For this review, take the finished solid that the model builds, in its own axes (mm). A direction names the side the tool comes from. Coordinates: 2 decimals unless noted, no trailing zeros. Write each loop counter-clockwise with the first axis right and the second up, starting at its lowest first coordinate (ties: lowest second). Pieces come first, ordered by that corner, then holes.
```python
from build123d import *

# Parameters (mm, degrees)
SKETCH_W             = 162
SKETCH_H             = 37
PAD_DEPTH            = 16
POCKET_DEPTH         = 18.501
POCKET_DEPTH_BACK    = -18.501
POCKET001_DEPTH      = 18.501
POCKET001_DEPTH_BACK = -18.501
POCKET002_DEPTH      = 18.501
POCKET002_DEPTH_BACK = -18.501
POCKET003_DEPTH      = 18.501
POCKET003_DEPTH_BACK = -18.501
POCKET004_DEPTH      = 18.501
POCKET004_DEPTH_BACK = -18.501
SKETCH004_W          = 31.24
SKETCH004_H          = 3.92
POCKET005_DEPTH      = 81.001
POCKET005_DEPTH_BACK = -81.001
SKETCH005_W          = 33.24
SKETCH005_H          = 1
POCKET006_DEPTH      = 81.001
POCKET006_DEPTH_BACK = -81.001


with BuildPart() as part:
    # Sketch → Pad (new body)
    with BuildSketch(Plane.XY):
        Rectangle(SKETCH_W, SKETCH_H)
    extrude(amount=PAD_DEPTH)

    # Sketch001 → Pocket (cut, two sides)
    with BuildSketch(Plane.XZ) as pocket_sk:
        Polygon((81, 16), (81, 9.14), (65, 9.14), (65, -1.45), (83.75, -1.45), (83.75, 16), align=None)
    extrude(amount=-POCKET_DEPTH, mode=Mode.SUBTRACT)
    extrude(pocket_sk.sketch, amount=-POCKET_DEPTH_BACK, mode=Mode.SUBTRACT)

    # MirroredSketch → Pocket001 (cut, two sides)
    with BuildSketch(Plane.XZ) as pocket001_sk:
        Polygon((-81, 16), (-81, 9.14), (-65, 9.14), (-65, -1.45), (-83.75, -1.45), (-83.75, 16), align=None)
    extrude(amount=-POCKET001_DEPTH, mode=Mode.SUBTRACT)
    extrude(pocket001_sk.sketch, amount=-POCKET001_DEPTH_BACK, mode=Mode.SUBTRACT)

    # Sketch002 → Pocket002 (cut, two sides)
    with BuildSketch(Plane.XZ) as pocket002_sk:
        with BuildLine():
            Line((57.5, 3.58), (57.5, -2.6))
            Line((57.5, -2.6), (46.5, -2.6))
            Line((46.5, -2.6), (46.5, 3.58))
            ThreePointArc((57.5, 3.58), (52, 9.08), (46.5, 3.58))
        make_face()
    extrude(amount=-POCKET002_DEPTH, mode=Mode.SUBTRACT)
    extrude(pocket002_sk.sketch, amount=-POCKET002_DEPTH_BACK, mode=Mode.SUBTRACT)

    # MirroredSketch001 → Pocket003 (cut, two sides)
    with BuildSketch(Plane.XZ) as pocket003_sk:
        with BuildLine():
            Line((-57.5, 3.58), (-57.5, -2.6))
            Line((-57.5, -2.6), (-46.5, -2.6))
            Line((-46.5, -2.6), (-46.5, 3.58))
            ThreePointArc((-46.5, 3.58), (-52, 9.08), (-57.5, 3.58))
        make_face()
    extrude(amount=-POCKET003_DEPTH, mode=Mode.SUBTRACT)
    extrude(pocket003_sk.sketch, amount=-POCKET003_DEPTH_BACK, mode=Mode.SUBTRACT)

    # Sketch003 → Pocket004 (cut, two sides)
    with BuildSketch(Plane.XZ) as pocket004_sk:
        with BuildLine():
            Line((-40.2, 4.78), (-40.2, -1.94))
            Line((-40.2, -1.94), (40.2, -1.94))
            Line((40.2, -1.94), (40.2, 4.78))
            ThreePointArc((40.2, 4.78), (39.707939, 5.967939), (38.52, 6.46))
            Line((38.52, 6.46), (-38.52, 6.46))
            ThreePointArc((-38.52, 6.46), (-39.707939, 5.967939), (-40.2, 4.78))
        make_face()
    extrude(amount=-POCKET004_DEPTH, mode=Mode.SUBTRACT)
    extrude(pocket004_sk.sketch, amount=-POCKET004_DEPTH_BACK, mode=Mode.SUBTRACT)

    # Sketch004 → Pocket005 (cut, two sides)
    with BuildSketch(Plane.YZ) as pocket005_sk:
        with Locations((0, 15.32)):
            Rectangle(SKETCH004_W, SKETCH004_H)
    extrude(amount=-POCKET005_DEPTH, mode=Mode.SUBTRACT)
    extrude(pocket005_sk.sketch, amount=-POCKET005_DEPTH_BACK, mode=Mode.SUBTRACT)

    # Sketch005 → Pocket006 (cut, two sides)
    with BuildSketch(Plane.YZ) as pocket006_sk:
        with Locations((0, 13.86)):
            Rectangle(SKETCH005_W, SKETCH005_H)
    extrude(amount=-POCKET006_DEPTH, mode=Mode.SUBTRACT)
    extrude(pocket006_sk.sketch, amount=-POCKET006_DEPTH_BACK, mode=Mode.SUBTRACT)


solid = part.part
```
Q1. Tool access review of faces 1 (the flat face through (-73, 0, 9.14)), 2 (the flat face through (65, 0, 5)), 3 (the flat face through (-1, -17, 16)), 4 (the flat face through (43, 0, 0)), 5 (the flat face through (-57.5, 0, 2)): name each direction out of +Z, -Z, +X, -X, +Y, -Y from which nothing blocks a thin tool from reaching the whole face with its end or side.
Ans:
face 1: -Z, -X, +Y, -Y
face 2: -Z, +X, +Y, -Y
face 3: +Z, +X, -X, +Y, -Y
face 4: -Z, +X, -X, +Y, -Y
face 5: -Z, +Y, -Y
Q2. Add section B-B (y = -7.5). State the section outline as (x, z) points, then the cut area to 3 significant figures.
Ans:
outline: (-81, 9.14) - (-65, 9.14) - (-65, 0) - (-57.5, 0) - (-57.5, 3.58) arc R5.5 cw to (-46.5, 3.58) - (-46.5, 0) - (-40.2, 0) - (-40.2, 4.78) arc R1.68 cw to (-38.52, 6.46) - (38.52, 6.46) arc R1.68 cw to (40.2, 4.78) - (40.2, 0) - (46.5, 0) - (46.5, 3.58) arc R5.5 cw to (57.5, 3.58) - (57.5, 0) - (65, 0) - (65, 9.14) - (81, 9.14) - (81, 13.36) - (-81, 13.36) - close
area: 1,180 mm2
Q3. For probe 1 along X at (y, z) = (14, 3.75); probe 2 along X at (y, z) = (0, 8); probe 3 along Y at (x, z) = (-40.5, 15), list the stretches that pass through material, from the lowest coordinate up.
Ans:
probe 1: x = -65 to -57.5, -46.5 to -40.2, 40.2 to 46.5, 57.5 to 65
probe 2: x = -65 to -55.27, -48.73 to 48.73, 55.27 to 65
probe 3: y = -18.5 to -15.62, 15.62 to 18.5
Q4. Draft analysis for pull direction X (two halves, no side actions). For faces 6 (the flat face through (1, 0, 6.46)), 7 (the flat face through (-65, 0, 5)), 8 (the flat face through (61, 0, 0)), state which applies: +X half, -X half, draft (parallel to the pull), parting line (faces both ways), or undercut.
Ans:
face 6: undercut
face 7: -X half
face 8: draft
Q5. Add section C-C (x = 63.5). State the section outline as (y, z) points, then the cut area to 3 significant figures.
Ans:
outline: (-18.5, 0) - (18.5, 0) - (18.5, 16) - (15.62, 16) - (15.62, 14.36) - (16.62, 14.36) - (16.62, 13.36) - (-16.62, 13.36) - (-16.62, 14.36) - (-15.62, 14.36) - (-15.62, 16) - (-18.5, 16) - close
area: 508 mm2
Q6. Add section A-A (x = -52). State the section outline as (y, z) points, then the cut area to 3 significant figures.
Ans:
outline: (-18.5, 9.08) - (18.5, 9.08) - (18.5, 16) - (15.62, 16) - (15.62, 14.36) - (16.62, 14.36) - (16.62, 13.36) - (-16.62, 13.36) - (-16.62, 14.36) - (-15.62, 14.36) - (-15.62, 16) - (-18.5, 16) - close
area: 172 mm2
Q7. Clearance check with flat-ended pins moving along their axes: pin 1 Ø2 at (y, z) = (2.5, 7.5) entering from +X; pin 2 Ø1.1 at (y, z) = (6.5, 2) entering from -X; pin 3 Ø8 at (x, y) = (-71, -4.5) entering from -Z; pin 4 Ø3 at (x, z) = (-8.5, 5) entering from +Y. State where each tip first meets the part, or that it passes through.
Ans:
pin 1: stops at x = 65
pin 2: stops at x = -65
pin 3: stops at z = 9.14
pin 4: stops at y = 18.5
